CAD build for the part. Positions are in the model's coordinates, mm. A direction names the side the tool comes from. Coordinates: 2 decimals unless noted, no trailing zeros. Write each loop counter-clockwise with the first axis right and the second up, starting at its lowest first coordinate (ties: lowest second). Pieces come first, ordered by that corner, then holes.
```python
from build123d import *

# Parameters (mm, degrees)
F3_W      = 38.1
F3_H      = 38.1
F4_DEPTH  = 38.1
F6_DEPTH  = 38.1
F8_DEPTH  = 38.1
F9_W      = 25.4
F9_H      = 7.62
F10_DEPTH = 38.1


with BuildPart() as f4:
    # F3 (on Front) → F4 (new body)
    with BuildSketch(Plane.XZ):
        with Locations((19.05, 19.05)):
            Rectangle(F3_W, F3_H)
    extrude(amount=-F4_DEPTH)

    # F5 (on offset) → F6 (cut)
    with BuildSketch(Plane.YZ.offset(38.1)):
        Polygon((31.75, 38.1), (6.35, 38.1), (11.43, 15.875), (16.51, 28.575), (21.59, 28.575), (26.67, 15.875), align=None)
        Polygon((0, 38.1), (0, 0), (6.35, 0), align=None)
        Polygon((19.05, 15.875), (12.7, 0), (25.4, 0), align=None)
        Polygon((38.1, 38.1), (31.75, 0), (38.1, 0), align=None)
    extrude(amount=-F6_DEPTH, mode=Mode.SUBTRACT)

    # F7 (on offset) → F8 (cut)
    with BuildSketch(Plane.XZ):
        Polygon((25.4, 38.1), (12.7, 38.1), (19.05, 23.510631), align=None)
        Polygon((6.35, 38.1), (0, 38.1), (0, 0), align=None)
        Polygon((11.43, 22.225), (6.35, 0), (31.75, 0), (26.67, 22.225), (21.59, 9.525), (16.51, 9.525), align=None)
        Polygon((31.75, 38.1), (38.1, 0), (38.1, 38.1), align=None)
    extrude(amount=-F8_DEPTH, mode=Mode.SUBTRACT)

    # F9 (on offset) → F10 (cut)
    with BuildSketch(Plane.XY.offset(38.1)):
        with Locations((25.4, 26.67)):
            Rectangle(F9_W, F9_H)
        with Locations((12.7, 11.43)):
            Rectangle(F9_W, F9_H)
    extrude(amount=-F10_DEPTH, mode=Mode.SUBTRACT)


solid = f4.part
```
Item 1: Saw through at D-D, the plane z = 20.5. State how many separate pieces and enclosed holes the cut face has, and give its area (3 significant figures).
Item 2: Saw through at A-A, the plane z = 34. Write the cut outline in (x, y).
Item 3: Which spindle directions (+Z, -Z, +X, -X, +Y, -Y) get a long thin tool onto all of the face, cutting with end or side? Do faces 4 (the flat face through (15.83, 4.6, 30.91)), 5 (the flat face through (16, 15.24, 18)), 6 (the flat face through (27, 19, 28.575)), 7 (the flat face through (9.49, 25.21, 13.74)). Say none if no direction does.
Item 4: Saw through at C-C, the plane z = 30. Write the cut outline in (x, y), and give its area (3 significant figures).
Item 5: Saw through at B-B, the plane y = 32.5. Write the cut outline in (x, z) (3 decimals).
Item 6: Wall check: line 1 along X through (y, z) = (34.5, 20); line 2 along Y through (x, z) = (14, 21); line 3 along Y through (x, z) = (33, 17.5). Give the ranges that are in metal, low to high.
Item 7: Two-plate mould, pull along X, no slides. Class faces 1 (the flat face through (12.7, 24, 21)), 2 (the flat face through (24.73, 5.72, 17.38)), 3 (the flat face through (33.2, 15.9, 8)): +X half, -X half, draft (parallel to the pull), parting line (faces both ways), or undercut.
Item 8: Flat gauge pins, fed straight in: pin 1 Ø1 at (x, y) = (18.5, 22.5) entering from -Z (3 decimals); pin 2 Ø12.5 at (x, z) = (31.5, 11.5) entering from -Y; pin 3 Ø8 at (y, z) = (31.5, 6.5) entering from +X; pin 4 Ø10 at (x, y) = (5, 27.5) entering from +Z. Where does each tip first touch, or does it go through?
Working result:
1. separate pieces: 9
1. enclosed holes: 0
1. area: 572 mm2
2. outline: (5.67, 0.68) - (14.48, 0.68) - (14.48, 7.29) - (5.67, 7.29) - close; (5.67, 30.81) - (14.48, 30.81) - (14.48, 37.42) - (5.67, 37.42) - close; (23.62, 0.68) - (32.43, 0.68) - (32.43, 7.29) - (23.62, 7.29) - close; (23.62, 30.81) - (32.43, 30.81) - (32.43, 37.42) - (23.62, 37.42) - close
3. face 4: +Z, +Y, -Y
3. face 5: +Z, -Z, -X
3. face 6: +Z, +X, -X
3. face 7: -Z, +Y, -Y
4. outline: (5, 1.35) - (16.23, 1.35) - (16.23, 7.62) - (5, 7.62) - close; (5, 29.9) - (12.7, 29.9) - (12.7, 30.48) - (16.23, 30.48) - (16.23, 36.75) - (5, 36.75) - close; (21.87, 1.35) - (33.1, 1.35) - (33.1, 8.2) - (25.4, 8.2) - (25.4, 7.62) - (21.87, 7.62) - close; (21.87, 30.48) - (33.1, 30.48) - (33.1, 36.75) - (21.87, 36.75) - close
4. area: 290 mm2
5. outline: (0.75, 4.5) - (7.379, 4.5) - (11.43, 22.225) - (16.51, 9.525) - (21.59, 9.525) - (26.67, 22.225) - (30.721, 4.5) - (37.35, 4.5) - (31.75, 38.1) - (25.4, 38.1) - (19.05, 23.511) - (12.7, 38.1) - (6.35, 38.1) - close
6. line 1: x = 3.33 to 10.92, 12.32 to 25.78, 27.18 to 34.77
6. line 2: y = 2.85 to 7.62, 15.24 to 22.86, 30.48 to 35.25
6. line 3: y = 3.43 to 11.06, 12.08 to 22.86, 30.48 to 34.67
7. face 1: +X half
7. face 2: undercut
7. face 3: draft
8. pin 1: stops at z = 9.525
8. pin 2: stops at y = 3.39
8. pin 3: stops at x = 37.68
8. pin 4: stops at z = 38.1
